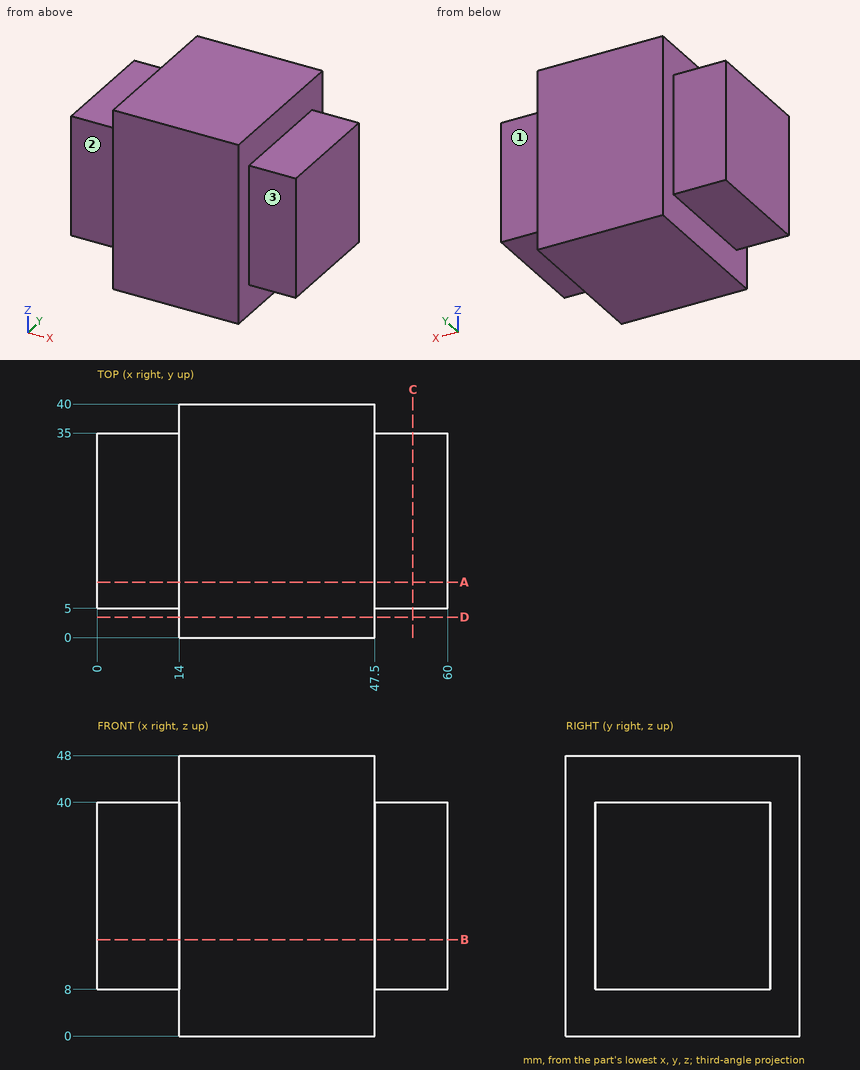
Design review of the part shown in the three views and the two pictorial views. Dimensions are in mm from the part's minimum x, y and z. A direction names the side the tool comes from. Round coordinates to 2 decimals unless told otherwise and drop trailing zeros. Loops run counter-clockwise (first coordinate to the right, second up) from the corner with the lowest first, then second, coordinate; pieces in that order, holes last.
1) Consider section D-D on y = 3.5. State the section outline as (x, z) points, then the cut area to 3 significant figures.
Values follow:
outline: (14, 0) - (47.5, 0) - (47.5, 48) - (14, 48) - close
area: 1,610 mm2
2) Tool access review of the marked faces 1, 2 and 3: name each direction out of +Z, -Z, +X, -X, +Y, -Y from which nothing blocks a thin tool from reaching the whole face with its end or side.
Values follow:
face 1: +Z, -Z, +X, +Y
face 2: +Z, -Z, -X, -Y
face 3: +Z, -Z, +X, -Y
3) Consider section B-B on z = 16.5. State the section outline as (x, y) points.
Values follow:
outline: (0, 5) - (14, 5) - (14, 0) - (47.5, 0) - (47.5, 5) - (60, 5) - (60, 35) - (47.5, 35) - (47.5, 40) - (14, 40) - (14, 35) - (0, 35) - close
4) Consider section C-C on x = 54. State the section outline as (y, z) points.
Values follow:
outline: (5, 8) - (35, 8) - (35, 40) - (5, 40) - close
5) Consider section A-A on y = 9.5. State the section outline as (x, z) points.
Values follow:
outline: (0, 8) - (14, 8) - (14, 0) - (47.5, 0) - (47.5, 8) - (60, 8) - (60, 40) - (47.5, 40) - (47.5, 48) - (14, 48) - (14, 40) - (0, 40) - close
6) Clearance check with flat-ended pins moving along their axes: P1, Ø10, axis at y = 26, z = 12.5, coming from the -X side; P2, Ø6, axis at x = 52, y = 16, coming from the -Z side; P3, Ø7, axis at x = 3.5, z = 24, coming from the +Y side; P4, Ø6, axis at x = 56, y = 18.5, coming from the +Z side. State where each tip first meets the part, or that it passes through.
Values follow:
P1: stops at x = 0
P2: stops at z = 8
P3: stops at y = 35
P4: stops at z = 40
7) Wall thickness on line 1 along X through (y, z) = (22.5, 42); line 2 along Z through (x, y) = (8.5, 11.5); line 3 along Y through (x, z) = (51, 13.5): over which ranges is each line inside the solid? List them lowest first.
Values follow:
line 1: x = 14 to 47.5
line 2: z = 8 to 40
line 3: y = 5 to 35
